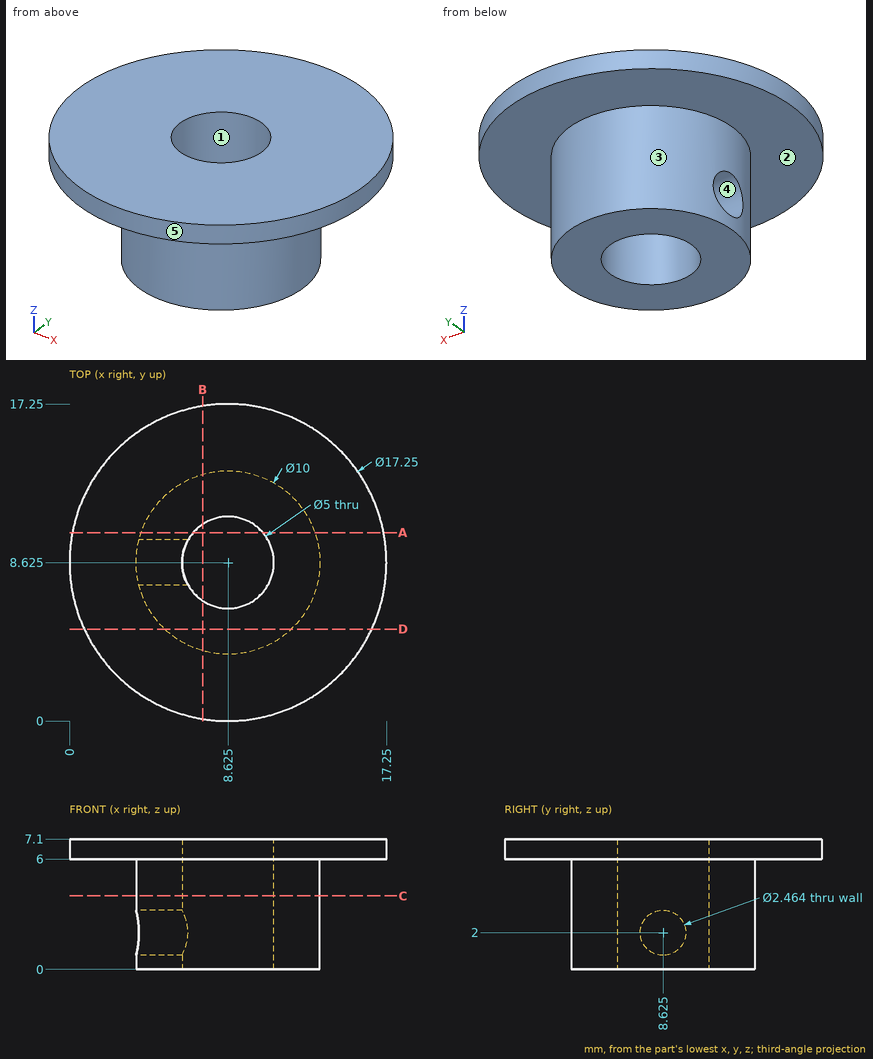
Design review of the part shown in the three views and the two pictorial views. Dimensions are in mm from the part's minimum x, y and z. A direction names the side the tool comes from. Give positions to 0.01 mm unless a question says otherwise; leave off trailing zeros. Write each loop counter-clockwise with the first axis right and the second up, starting at its lowest first coordinate (ties: lowest second). Pieces come first, ordered by that corner, then holes. Notation, with made-up numbers: M 53.5,61 L 74.5,61 A23 ccw 74.5,89 Z; hole C -19.5,67 d8. An arc over 180 degrees is marked long. One line per question, with ' | ' between items. Start each with the question number.
Item 1: We need section A-A on y = 10.25. Write out the cut boundary in (x, z) (1 decimal), plus the area to 3 significant figures.
Item 2: Draft analysis for pull direction X (two halves, no side actions). For the marked faces 1, 2 and 3, state which applies: released by +X, released by -X, zero draft, split by the parting line, or undercut.
Item 3: For pin 1 (4 mm diameter, centred on x = 15.5, y = 11, fed in from -Z); pin 2 (1 mm diameter, centred on x = 9, z = 4, fed in from +Y) (3 decimals); pin 3 (4 mm diameter, centred on y = 8.625, z = 2, fed in from +X) (3 decimals), all flat-tipped, find the tip position at first contact; note any pin that passes through.
Item 4: We need section C-C on z = 4. Write out the cut boundary in (x, y) (3 decimals).
Item 5: For the marked faces 4 and 5, list the 3-axis set-ups (+Z, -Z, +X, -X, +Y, -Y) from which the entire face can be reached by the end or side of a thin tool; tool diameter is ignored.
Item 6: We need section D-D on y = 5. Write out the cut boundary in (x, z).
Item 7: We need section B-B on x = 7.25. Write out the cut boundary in (y, z).
Item 8: Wall thickness on line 1 (Z direction, x = 2.75, y = 4.75); line 2 (X direction, y = 10, z = 4); line 3 (X direction, y = 8.75, z = 3.5): over which ranges is each line inside the solid? List them lowest first. Write a range as from..to.
Results found:
1) outline: M 0.2,6 L 3.9,6 L 3.9,0 L 6.7,0 L 6.7,7.1 L 0.2,7.1 Z; M 10.5,0 L 13.4,0 L 13.4,6 L 17.1,6 L 17.1,7.1 L 10.5,7.1 Z | area: 48.4 mm2
2) face 1: undercut | face 2: zero draft | face 3: split by the parting line
3) pin 1: stops at z = 6 | pin 2: stops at y = 13.625 | pin 3: stops at x = 13.625
4) outline: C 8.625,8.625 d10; hole C 8.625,8.625 d5
5) face 4: -X | face 5: +Z, -Z
6) outline: M 0.8,6 L 5.18,6 L 5.18,0 L 12.07,0 L 12.07,6 L 16.45,6 L 16.45,7.1 L 0.8,7.1 Z
7) outline: M 0.11,6 L 3.82,6 L 3.82,0 L 6.54,0 L 6.54,7.1 L 0.11,7.1 Z; M 10.71,0 L 13.43,0 L 13.43,6 L 17.14,6 L 17.14,7.1 L 10.71,7.1 Z
8) line 1: z = 6..7.1 | line 2: x = 3.82..6.54, 10.71..13.43 | line 3: x = 3.63..6.13, 11.12..13.62
